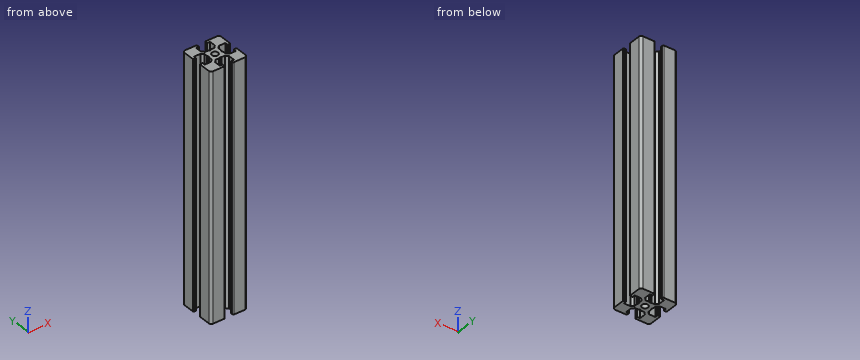
Autodesk Inventor part; units mm, degrees
ref_plane "YZ Plane" through (0, 0, 0) normal (1, 0, 0) x (0, 1, 0)
ref_plane "XZ Plane" through (0, 0, 0) normal (0, 1, 0) x (-1, 0, 0)
ref_plane "XY Plane" through (0, 0, 0) normal (0, 0, 1) x (1, 0, 0)
sketch "Sketch_1" plane through (0, 0, 0) normal (0, 0, 1) x (1, 0, 0)
  arc A0 (-7.5, 2) -> (-7.2, 1.7) centre (-7.2, 2) ccw
  line L0 (-7.2, 1.7) -> (-6.4, 1.7)
  line L1 (-6.4, 1.7) -> (-6.4, 2.85)
  line L2 (-6.4, 2.85) -> (-3.8, 2.85)
  line L3 (-3.8, 2.85) -> (-2.8, 1.85)
  line L4 (-2.8, 1.85) -> (-2.8, 0.5196)
  line L5 (-2.8, 0.5196) -> (-2.5, 0)
  line L6 (-2.5, 0) -> (-2.8, -0.5196)
  line L7 (-2.8, -0.5196) -> (-2.8, -1.85)
  line L8 (-2.8, -1.85) -> (-3.8, -2.85)
  line L9 (-3.8, -2.85) -> (-6.4, -2.85)
  line L10 (-6.4, -2.85) -> (-6.4, -1.7)
  line L11 (-6.4, -1.7) -> (-7.2, -1.7)
  arc A1 (-7.2, -1.7) -> (-7.5, -2) centre (-7.2, -2) ccw
  line L12 (-7.5, -2) -> (-7.5, -6.5)
  arc A2 (-7.5, -6.5) -> (-6.5, -7.5) centre (-6.5, -6.5) ccw
  line L13 (-6.5, -7.5) -> (-2, -7.5)
  arc A3 (-2, -7.5) -> (-1.7, -7.2) centre (-2, -7.2) ccw
  line L14 (-1.7, -7.2) -> (-1.7, -6.4)
  line L15 (-1.7, -6.4) -> (-2.85, -6.4)
  line L16 (-2.85, -6.4) -> (-2.85, -3.8)
  line L17 (-2.85, -3.8) -> (-1.85, -2.8)
  line L18 (-1.85, -2.8) -> (-0.5196, -2.8)
  line L19 (-0.5196, -2.8) -> (0, -2.5)
  line L20 (0, -2.5) -> (0.5196, -2.8)
  line L21 (0.5196, -2.8) -> (1.85, -2.8)
  line L22 (1.85, -2.8) -> (2.85, -3.8)
  line L23 (2.85, -3.8) -> (2.85, -6.4)
  line L24 (2.85, -6.4) -> (1.7, -6.4)
  line L25 (1.7, -6.4) -> (1.7, -7.2)
  arc A4 (1.7, -7.2) -> (2, -7.5) centre (2, -7.2) ccw
  line L26 (2, -7.5) -> (6.5, -7.5)
  arc A5 (6.5, -7.5) -> (7.5, -6.5) centre (6.5, -6.5) ccw
  line L27 (7.5, -6.5) -> (7.5, -2)
  arc A6 (7.5, -2) -> (7.2, -1.7) centre (7.2, -2) ccw
  line L28 (7.2, -1.7) -> (6.4, -1.7)
  line L29 (6.4, -1.7) -> (6.4, -2.85)
  line L30 (6.4, -2.85) -> (3.8, -2.85)
  line L31 (3.8, -2.85) -> (2.8, -1.85)
  line L32 (2.8, -1.85) -> (2.8, -0.5196)
  line L33 (2.8, -0.5196) -> (2.5, 0)
  line L34 (2.5, 0) -> (2.8, 0.5196)
  line L35 (2.8, 0.5196) -> (2.8, 1.85)
  line L36 (2.8, 1.85) -> (3.8, 2.85)
  line L37 (3.8, 2.85) -> (6.4, 2.85)
  line L38 (6.4, 2.85) -> (6.4, 1.7)
  line L39 (6.4, 1.7) -> (7.2, 1.7)
  arc A7 (7.2, 1.7) -> (7.5, 2) centre (7.2, 2) ccw
  line L40 (7.5, 2) -> (7.5, 6.5)
  arc A8 (7.5, 6.5) -> (6.5, 7.5) centre (6.5, 6.5) ccw
  line L41 (6.5, 7.5) -> (2, 7.5)
  arc A9 (2, 7.5) -> (1.7, 7.2) centre (2, 7.2) ccw
  line L42 (1.7, 7.2) -> (1.7, 6.4)
  line L43 (1.7, 6.4) -> (2.85, 6.4)
  line L44 (2.85, 6.4) -> (2.85, 3.8)
  line L45 (2.85, 3.8) -> (1.85, 2.8)
  line L46 (1.85, 2.8) -> (0.5196, 2.8)
  line L47 (0.5196, 2.8) -> (0, 2.5)
  line L48 (0, 2.5) -> (-0.5196, 2.8)
  line L49 (-0.5196, 2.8) -> (-1.85, 2.8)
  line L50 (-1.85, 2.8) -> (-2.85, 3.8)
  line L51 (-2.85, 3.8) -> (-2.85, 6.4)
  line L52 (-2.85, 6.4) -> (-1.7, 6.4)
  line L53 (-1.7, 6.4) -> (-1.7, 7.2)
  arc A10 (-1.7, 7.2) -> (-2, 7.5) centre (-2, 7.2) ccw
  line L54 (-2, 7.5) -> (-6.5, 7.5)
  arc A11 (-6.5, 7.5) -> (-7.5, 6.5) centre (-6.5, 6.5) ccw
  line L55 (-7.5, 6.5) -> (-7.5, 2)
  circle A12 centre (0, 0) radius 1.25
extrude "Extrusion1" add sketch "Sketch_1" along normal blind 100
equation "\"d0\" = L"
equation "\"L\" = 100"
properties part number "HFS3-1515-100"
Geometry: final body of the model. Coordinates: model frame, mm. Coordinates: 2 decimals unless noted, no trailing zeros. Write each loop counter-clockwise with the first axis right and the second up, starting at its lowest first coordinate (ties: lowest second). Pieces come first, ordered by that corner, then holes. Notation, with made-up numbers: M -7,41 L 44,41 A22 ccw 44,68 Z; hole C 4.25,-18.75 d2. An arc over 180 degrees is marked long. Use CSV: the item, a comma, the result in double quotes. Start each with the question number.
1. Ray query, probe 1 along Y at (x, z) = (0, 73.5); probe 2 along X at (y, z) = (-2.75, 32). Return the intervals inside material, ascending.
2. Cut plane A-A on x = -5.5. Return the cut outline in (y, z).
3. First-contact query: P1, Ø1.1, axis at y = -1, z = 62.5, coming from the -X side; P2, Ø0.7, axis at y = 1.5, z = 69.5, coming from the -X side; P3, Ø2, axis at x = 0, y = 0, coming from the +Z side. Flat tips, straight axial feed; report the tip coordinate or a pass-through.
Entries:
1,probe 1,"-2.5 to -1.25, 1.25 to 2.5"
1,probe 2,"-7.5 to -6.4, -3.7 to -0.43, 0.43 to 3.7, 6.4 to 7.5"
2,outline,"M -7.5,0 L -2.85,0 L -2.85,100 L -7.5,100 Z; M 2.85,0 L 7.5,0 L 7.5,100 L 2.85,100 Z"
3,P1,"x = -2.8"
3,P2,"x = -7.46"
3,P3,"through"
